Check sheet for the modelled part. Datum: model origin and axes. Units: mm. Round coordinates to 2 decimals unless told otherwise and drop trailing zeros. Write each loop counter-clockwise with the first axis right and the second up, starting at its lowest first coordinate (ties: lowest second). Pieces come first, ordered by that corner, then holes. Notation, with made-up numbers: (34, 81.5) -> (56, 81.5) arc R12 ccw to (56, 87.5) -> close; hole circle Ø10 at (-36, 62.25). An arc over 180 degrees is marked (long way). Use one line per item in the form item = value. Start each with the question number.
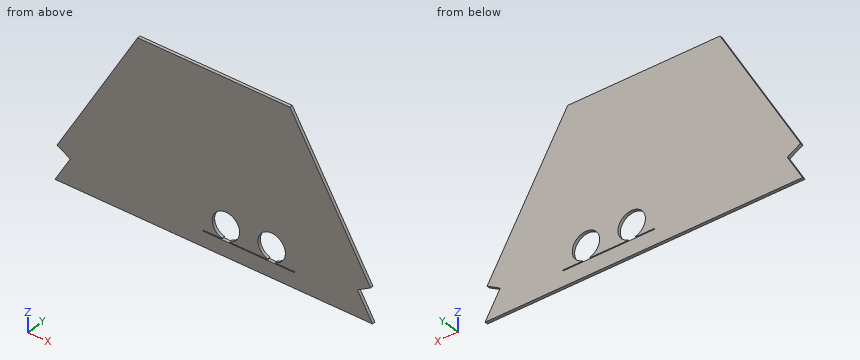
```python
from build123d import *

# Parameters (mm, degrees)
BOSS_EXTRUDE1_DEPTH = 10
CUT_EXTRUDE6_DEPTH  = 10


with BuildPart() as part:
    # Sketch1 → Boss-Extrude1 (new body)
    with BuildSketch(Plane(origin=(0, 0, 0), x_dir=(1, 0, 0), z_dir=(0, 1, 0))):
        Polygon((-271.133729811, 569.617395678), (771.133729811, 569.617395678), (721.133729811, 483.014855299), (764.435, 458.014855299), (500, 0), (0, 0), (-264.435, 458.014855299), (-221.133729811, 483.014855299), align=None)
    extrude(amount=BOSS_EXTRUDE1_DEPTH)

    # Sketch2 → Cut-Extrude6 (cut)
    with BuildSketch(Plane(origin=(0, 0, 0), x_dir=(-1, 0, 0), z_dir=(0, -1, 0))):
        with BuildLine():
            Line((-514.883729811, 519.62), (-514.883729811, 516.62))
            Line((-514.883729811, 516.62), (-452.38, 516.62))
            Line((-452.38, 516.62), (-452.38, 514.849041164))
            ThreePointArc((-452.38, 514.849041164), (-439.88, 426.62), (-427.38, 514.849041164))
            Line((-427.38, 514.849041164), (-427.38, 516.62))
            Line((-427.38, 516.62), (-302.38, 516.62))
            Line((-302.38, 516.62), (-302.38, 514.849041164))
            ThreePointArc((-302.38, 514.849041164), (-289.88, 426.62), (-277.38, 514.849041164))
            Line((-277.38, 514.849041164), (-277.38, 516.62))
            Line((-277.38, 516.62), (-214.883729811, 516.62))
            Line((-214.883729811, 516.62), (-214.883729811, 519.62))
            Line((-214.883729811, 519.62), (-514.883729811, 519.62))
        make_face()
    extrude(amount=-CUT_EXTRUDE6_DEPTH, mode=Mode.SUBTRACT)


solid = part.part
```
1. Scan lines: probe 1 along Z at (x, y) = (289.88, 7.75); probe 2 along X at (y, z) = (5.75, -443.5); probe 3 along X at (y, z) = (2.75, -471.62). Record each from-to range of solid material in increasing order.
2. Sectioned sample at A-A (x = 439.88). Enter the section's corners in (y, z), and give its area (3 significant figures).
3. Depth check by flat-ended pin: pin 1 (5 mm diameter, centred on y = 5, z = -210, fed in from -X); pin 2 (3 mm diameter, centred on y = 7.5, z = -172.5, fed in from +X); pin 3 (0.9 mm diameter, centred on y = 6, z = -516, fed in from +X). Enter the tip coordinate at first touch or a pass-through.
4. Sectioned sample at C-C (z = -471.62). Enter the section's corners in (x, y).
5. Sectioned sample at D-D (x = 640). Enter the section's corners in (y, z).
6. Sectioned sample at B-B (y = 1.5). Enter the section's corners in (x, z) (3 decimals), and give its area (3 significant figures).
Returned:
q1.probe_1 = -569.62 to -519.62, -426.62 to 0
q1.probe_2 = -256.05 to 254.75, 325.01 to 404.75, 475.01 to 756.05
q1.probe_3 = -240.87 to 244.88, 334.88 to 394.88, 484.88 to 740.87
q2.outline = (0, -569.62) -> (10, -569.62) -> (10, -519.62) -> (0, -519.62) -> close; (0, -426.62) -> (10, -426.62) -> (10, 0) -> (0, 0) -> close
q2.area = 4,770 mm^2
q3.pin_1 = -122.69
q3.pin_2 = 600.46
q3.pin_3 = 740.44
q4.outline = (-240.87, 0) -> (244.88, 0) -> (244.88, 10) -> (-240.87, 10) -> close; (334.88, 0) -> (394.88, 0) -> (394.88, 10) -> (334.88, 10) -> close; (484.88, 0) -> (740.87, 0) -> (740.87, 10) -> (484.88, 10) -> close
q5.outline = (0, -569.62) -> (10, -569.62) -> (10, -242.49) -> (0, -242.49) -> close
q6.outline = (-271.134, -569.617) -> (771.134, -569.617) -> (721.134, -483.015) -> (764.435, -458.015) -> (500, 0) -> (0, 0) -> (-264.435, -458.015) -> (-221.134, -483.015) -> close; hole (214.884, -519.62) -> (514.884, -519.62) -> (514.884, -516.62) -> (452.38, -516.62) -> (452.38, -514.849) arc R45 ccw (long way) to (427.38, -514.849) -> (427.38, -516.62) -> (302.38, -516.62) -> (302.38, -514.849) arc R45 ccw (long way) to (277.38, -514.849) -> (277.38, -516.62) -> (214.884, -516.62) -> close
q6.area = 447,000 mm^2
